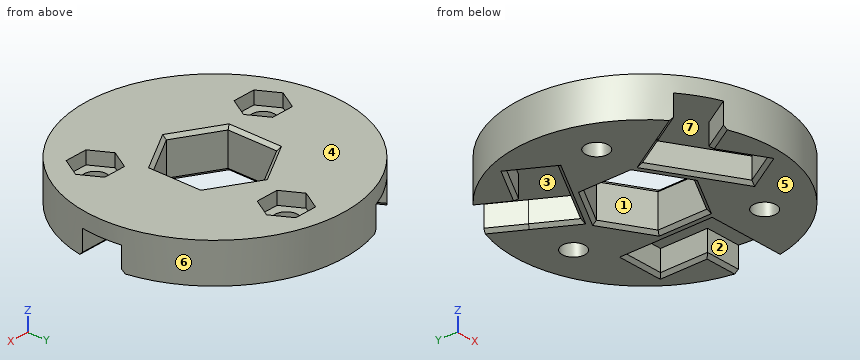
Autodesk Fusion 360 part; units mm, degrees
sketch "Esquisse1" plane through (0, 0, 0) normal (0, 0, 1) x (1, 0, 0)
  circle A0 centre (0, 0) radius 20
  line L0 (19.7661, -3.05) -> (8.2661, -3.05)
  line L1 (8.2661, -3.05) -> (8.2661, 3.1)
  line L2 (14.3661, 3.05) -> (19.7661, 3.05)
  line L3 (8.2661, -3.05) -> (14.4604, -3.05)
  line L4 (14.3661, 10.35) -> (8.2661, 10.35)
  line L5 (8.2661, 10.35) -> (8.2661, -3.05)
  line L6 (0, 0) -> (29, 0) construction
  line L7 (14.3661, 3.05) -> (14.3661, 10.35)
  line L8 (-9.8244, 10.9164) -> (-16.1464, 7.2664)
  line L9 (-16.1464, 7.2664) -> (-13.0964, 1.9836)
  line L10 (-13.0964, 1.9836) -> (-1.4917, 8.6836)
  line L11 (-1.4917, 8.6836) -> (-4.5888, 14.0481)
  line L12 (-7.2417, 18.6429) -> (-1.4917, 8.6836)
  line L13 (-9.8244, 10.9164) -> (-12.5244, 15.5929)
  line L14 (-4.5417, -13.9664) -> (1.7803, -17.6164)
  line L15 (1.7803, -17.6164) -> (4.8303, -12.3336)
  line L16 (4.8303, -12.3336) -> (-6.7744, -5.6336)
  line L17 (-6.7744, -5.6336) -> (-9.8716, -10.9981)
  line L18 (-12.5244, -15.5929) -> (-6.7744, -5.6336)
  line L19 (-4.5417, -13.9664) -> (-7.2417, -18.6429)
  circle A1 centre (2.9108, 13.6941) radius 1.75
  line L20 (0, 0) -> (2.9108, 13.6941) construction
  circle A2 centre (-13.3148, -4.3262) radius 1.75
  circle A3 centre (10.404, -9.3678) radius 1.75
  line L21 (0, 7.5633) -> (-6.55, 3.7816)
  line L22 (-6.55, 3.7816) -> (-6.55, -3.7816)
  line L23 (-6.55, -3.7816) -> (0, -7.5633)
  line L24 (0, -7.5633) -> (6.55, -3.7816)
  line L25 (6.55, -3.7816) -> (6.55, 3.7816)
  line L26 (6.55, 3.7816) -> (0, 7.5633)
  dimension "d1" = 40
  dimension "d2" = 6.1
  dimension "d3" = 11.5
  dimension "d6" = 6.1
  dimension "d7" = 3.05
  dimension "d8" = 13.4
  dimension "d10" = 360
  dimension "d16" = 3.5
  dimension "d17" = 78
  dimension "d19" = 360
  dimension "d21" = 14
  dimension "d25" = 6.55
extrude "Extrusion1" add sketch "Esquisse1" along normal blind 6.1 contours A0 L0 L1 L2 L3 L4 L5 L7 | A0 L0 L1 L2 L3 L4 L5 L7 L8 L9 L10 L11 L12 L13 L14 L15 L16 L17 L18 L19 | A0 L8 L9 L10 L11 L12 L13 | A0 L14 L15 L16 L17 L18 L19 | A1 | A2 | A3 | L21 L22 L23 L24 L25 L26
extrude "Extrusion2" cut sketch "Esquisse1" along normal blind 3.7 contours A0 L0 L1 L2 L3 L4 L5 L7 | A0 L8 L9 L10 L11 L12 L13 | A0 L14 L15 L16 L17 L18 L19
extrude "Extrusion3" cut sketch "Esquisse1" along normal blind 6.1 contours A1 | A2 | A3
chamfer "Chanfrein1" distance 0.5 angle 45 15 edges at (-4.3667, 13.6633, 0) (-11.1744, 13.2546, 0) (-12.9854, 9.0914, 0) (-14.6214, 4.625, 0) (-7.294, 5.3336, 0) (-9.6494, -10.6133, 0) (-0.972, -8.9836, 0) (-5.8917, -16.3046, 0) (-1.3807, -15.7914, 0) (3.3053, -14.975, 0) (8.2661, 3.65, 0) (14.0161, -3.05, 0) (17.0661, 3.05, 0) (14.3661, 6.7, 0) (11.3161, 10.35, 0)
extrude "Extrusion4" cut sketch "Esquisse1" along normal blind 6.1 contours L21 L22 L23 L24 L25 L26
chamfer "Chanfrein2" distance 0.5 angle 45 6 edges at (-3.275, -5.6725, 6.1) (-6.55, 0, 6.1) (-3.275, 5.6725, 6.1) (3.275, 5.6725, 6.1) (6.55, 0, 6.1) (3.275, -5.6725, 6.1)
chamfer "Chanfrein3" distance 0.5 angle 45 6 edges at (-6.55, 0, 0) (-3.275, -5.6725, 0) (3.275, -5.6725, 0) (6.55, 0, 0) (3.275, 5.6725, 0) (-3.275, 5.6725, 0)
sketch "Esquisse3" plane through (0, 0, 6.1) normal (0, 0, 1) x (-1, 0, 0)
  circle A0 centre (0, 0) radius 20
  circle A1 centre (-2.9108, -13.6941) radius 1.75
  circle A2 centre (13.3148, 4.3262) radius 1.75
  circle A3 centre (-10.404, 9.3678) radius 1.75
  line L0 (-7.05, -4.0703) -> (-7.05, 4.0703)
  line L1 (-7.05, 4.0703) -> (0, 8.1406)
  line L2 (0, 8.1406) -> (7.05, 4.0703)
  line L3 (7.05, 4.0703) -> (7.05, -4.0703)
  line L4 (7.05, -4.0703) -> (0, -8.1406)
  line L5 (0, -8.1406) -> (-7.05, -4.0703)
  line L6 (-4.6428, -10.6941) -> (-6.3749, -13.6941)
  line L7 (-6.3749, -13.6941) -> (-4.6428, -16.6941)
  line L8 (-4.6428, -16.6941) -> (-1.1787, -16.6941)
  line L9 (-1.1787, -16.6941) -> (0.5533, -13.6941)
  line L10 (0.5533, -13.6941) -> (-1.1787, -10.6941)
  line L11 (-1.1787, -10.6941) -> (-4.6428, -10.6941)
  line L12 (9.8507, 4.3262) -> (11.5827, 1.3262)
  line L13 (11.5827, 7.3262) -> (9.8507, 4.3262)
  line L14 (15.0468, 7.3262) -> (11.5827, 7.3262)
  line L15 (16.7789, 4.3262) -> (15.0468, 7.3262)
  line L16 (15.0468, 1.3262) -> (16.7789, 4.3262)
  line L17 (11.5827, 1.3262) -> (15.0468, 1.3262)
  line L18 (-8.672, 6.3678) -> (-6.9399, 9.3678)
  line L19 (-12.1361, 6.3678) -> (-8.672, 6.3678)
  line L20 (-13.8681, 9.3678) -> (-12.1361, 6.3678)
  line L21 (-12.1361, 12.3678) -> (-13.8681, 9.3678)
  line L22 (-8.672, 12.3678) -> (-12.1361, 12.3678)
  line L23 (-6.9399, 9.3678) -> (-8.672, 12.3678)
  point P0 (-2.9108, -13.6941)
  dimension "d30" = 3
  dimension "d32" = 360
extrude "Extrusion5" cut sketch "Esquisse3" against normal blind 2 contours L6 L7 L8 L9 L10 L11 | L12 L13 L14 L15 L16 L17 | L18 L19 L20 L21 L22 L23
equation "d6 = d2"
equation "d7 = d2 / 2"
Geometry check sheet. Reference: the model listing, model coordinates, mm. Face numbers are marked on the shaded views. A direction names the side the tool comes from. Round coordinates to 2 decimals unless told otherwise and drop trailing zeros. Loops run counter-clockwise (first coordinate to the right, second up) from the corner with the lowest first, then second, coordinate; pieces in that order, holes last.
Item 1: Access from +Z, -Z, +X, -X, +Y, -Y to the whole of each face (thin tool, end or side, straight path). Record for the marked faces 1, 2, 3 and 4.
Item 2: Cross-section at B-B on y = 0. Record the boundary of the cut face in (x, z).
Item 3: Cross-section at A-A on z = 4.75. Record the boundary of the cut face in (x, y), then the cut area to 3 significant figures.
Item 4: Cross-section at C-C on x = -14.5. Record the boundary of the cut face in (y, z), then the cut area to 3 significant figures.
Item 5: Mould release check, pull along X, two halves, no side actions. Record for the marked faces 5, 6 and 7: pulls with the +X half, pulls with the -X half, needs draft (parallel to the pull), parting line crosses it, or undercut.
Item 6: Cross-section at D-D on z = 2.25. Count the separate pieces of the cut face and the enclosed holes in it, then the cut area to 3 significant figures.
Item 7: Gauge pin test, flat ends, axial feed: pin 1 (4.5 mm diameter, centred on x = 10.4, y = -9.37, fed in from +Z); pin 2 (4 mm diameter, centred on x = -6, y = -10, fed in from -Z); pin 3 (1.5 mm diameter, centred on y = 6.5, z = 5, fed in from +X). Record the tip position at first contact, or that the pin passes through.
Item 8: Thickness scan on line 1 (X direction, y = 5, z = 1.75); line 2 (X direction, y = -15.5, z = 0.75); line 3 (Y direction, x = 5, z = 5). Record the ranges inside material, lowest first.
Answer sheet:
1. face 1: +Z, -Z
1. face 2: -Z, +X
1. face 3: -Z
1. face 4: +Z, +X, -X, +Y, -Y
2. outline: (-20, 0) - (-7.05, 0) - (-6.55, 0.5) - (-6.55, 5.6) - (-7.05, 6.1) - (-20, 6.1) - close; (6.55, 0.5) - (7.05, 0) - (7.77, 0) - (8.27, 0.5) - (8.27, 3.7) - (20, 3.7) - (20, 6.1) - (7.05, 6.1) - (6.55, 5.6) - close
3. outline: circle Ø40 at (0, 0); hole (-16.78, -4.33) - (-15.05, -7.33) - (-11.58, -7.33) - (-9.85, -4.33) - (-11.58, -1.33) - (-15.05, -1.33) - close; hole (-6.55, -3.78) - (0, -7.56) - (6.55, -3.78) - (6.55, 3.78) - (0, 7.56) - (-6.55, 3.78) - close; hole (-0.55, 13.69) - (1.18, 10.69) - (4.64, 10.69) - (6.37, 13.69) - (4.64, 16.69) - (1.18, 16.69) - close; hole (6.94, -9.37) - (8.67, -12.37) - (12.14, -12.37) - (13.87, -9.37) - (12.14, -6.37) - (8.67, -6.37) - close
3. area: 1,010 mm2
4. outline: (-13.77, 0) - (-5.61, 0) - (-5.61, 4.1) - (-7.33, 4.1) - (-7.33, 6.1) - (-13.77, 6.1) - close; (-3.04, 0) - (3.41, 0) - (4.41, 0.5) - (4.41, 3.7) - (8.22, 3.7) - (8.22, 0.5) - (8.79, 0) - (13.77, 0) - (13.77, 6.1) - (-1.33, 6.1) - (-1.33, 4.1) - (-3.04, 4.1) - close
4. area: 131 mm2
5. face 5: needs draft
5. face 6: parting line crosses it
5. face 7: undercut
6. separate pieces: 1
6. enclosed holes: 4
6. area: 732 mm2
7. pin 1: stops at z = 4.1
7. pin 2: stops at z = 3.7
7. pin 3: stops at x = 19.16
8. line 1: x = -19.36 to -14.84, -7.87 to -4.44, 4.44 to 8.27, 14.37 to 19.36
8. line 2: x = -12.64 to -12.47, -5.43 to -1.89, 3 to 12.64
8. line 3: y = -19.36 to -4.68, 4.68 to 11.31, 16.08 to 19.36
